Input: dimensioned drawing with shaded views. Units: mm. Origin: part minimum x, y, z. Round coordinates to 2 decimals unless told otherwise and drop trailing zeros. Write each loop counter-clockwise with the first axis right and the second up, starting at its lowest first coordinate (ties: lowest second). Pieces come first, ordered by that corner, then holes. Notation, with made-up numbers: (31.25, 52.5) - (37.25, 52.5) arc R18 cw to (37.25, 60.5) - close; hole circle Ø4 at (-15, 31). An arc over 180 degrees is marked (long way). Write item = value, one per line. Start each with the question number.
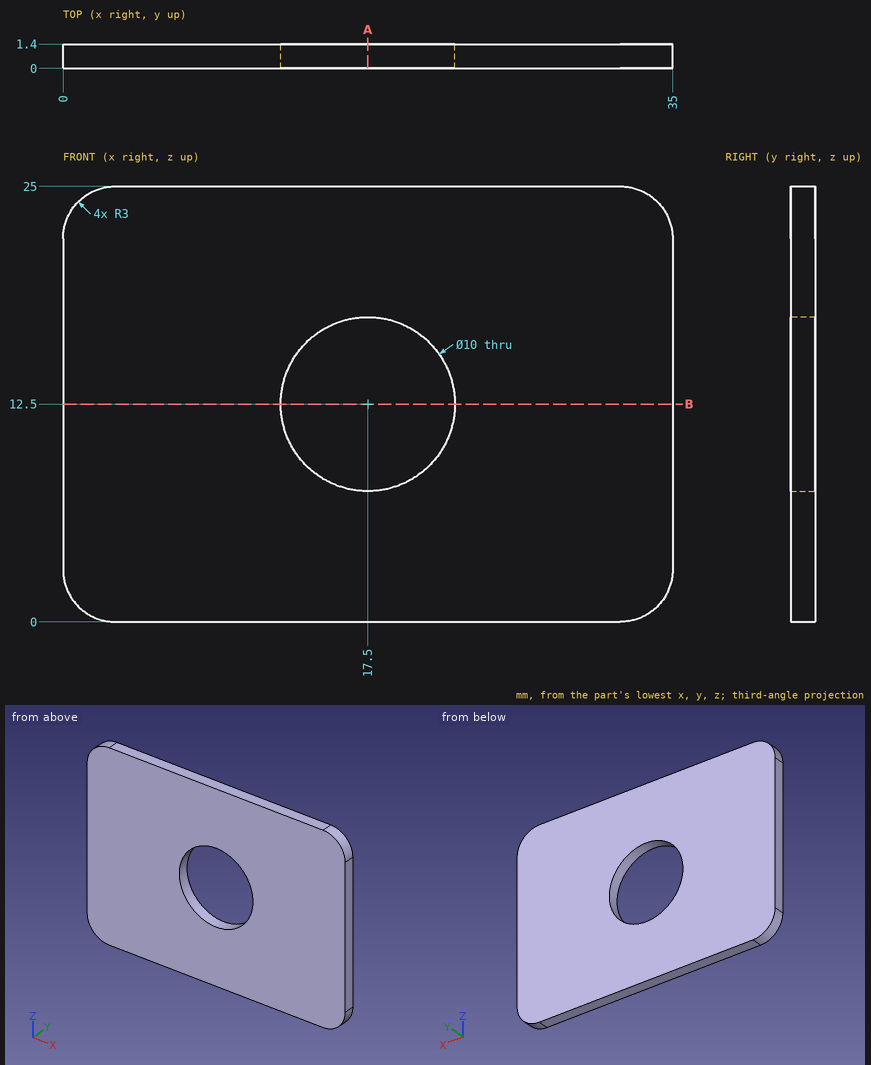
(1) Section B-B (z = 12.5). Return the cut outline in (x, y), plus the area to 3 significant figures.
(2) Contact query for flat-ended pins moving along their axis: P1, Ø9, axis at x = 17.5, z = 12.5, coming from the -Y side; P2, Ø8, axis at x = 7.5, z = 5.5, coming from the -Y side. Output: stop coordinate, or through.
(3) Ray query, L1, parallel to X at y = 0.45, z = 12.5; L2, parallel to Z at x = 21, y = 0.6; L3, parallel to X at y = 1.2, z = 9. Return the intervals inside material, ascending. Write a range as from..to.
(4) Section A-A (x = 17.5). Return the cut outline in (y, z), plus the area to 3 significant figures.
Solution:
q1.outline = (0, 0) - (12.5, 0) - (12.5, 1.4) - (0, 1.4) - close; (22.5, 0) - (35, 0) - (35, 1.4) - (22.5, 1.4) - close
q1.area = 35.0 mm^2
q2.P1 = through
q2.P2 = 0
q3.L1 = 0..12.5, 22.5..35
q3.L2 = 0..8.93, 16.07..25
q3.L3 = 0..13.93, 21.07..35
q4.outline = (0, 0) - (1.4, 0) - (1.4, 7.5) - (0, 7.5) - close; (0, 17.5) - (1.4, 17.5) - (1.4, 25) - (0, 25) - close
q4.area = 21.0 mm^2
